Source: CAD feature listing. Evaluate the final solid. Frame: model axes, mm. Face numbers are marked on the shaded views. A direction names the side the tool comes from. Give positions to 0.01 mm unless a question says otherwise; leave off trailing zeros. Loops run counter-clockwise (first coordinate to the right, second up) from the corner with the lowest first, then second, coordinate; pieces in that order, holes last. Notation, with made-up numbers: (47, 41.5) -> (57, 41.5) arc R19 cw to (57, 55.5) -> close; hole circle Ø9 at (-40, 30.25). An arc over 180 degrees is marked (long way). Return JSON: item names as keys, results as strings. Group by question number.
(1) Draft query along Y for the marked faces 1, 2 and 3. Return one class per face: released by +Y, released by -Y, zero draft, split by the parting line, or undercut.
(2) Cut plane A-A on z = 14. Return loops of the section in (x, y), then the cut area to 3 significant figures.
(3) Pin query (flat end, axial travel): pin 1 (4 mm diameter, centred on x = 77, y = 83.5, fed in from -Z); pin 2 (10 mm diameter, centred on x = -167, z = 35.5, fed in from -Y); pin 3 (21 mm diameter, centred on y = -2, z = 13, fed in from -X); pin 4 (3 mm diameter, centred on x = -65, y = -16, fed in from -Z). Return the tip coordinate at first contact, or that it passes through.
(4) Cut plane C-C on x = -182. Return loops of the section in (y, z).
(5) Ray query, line 1 (Y direction, x = 21, z = 6); line 2 (Z direction, x = 36, y = -54); line 3 (Y direction, x = -1, z = 8). Return the intervals inside material, ascending. Write a range as from..to.
(6) Cut plane B-B on x = 12. Return loops of the section in (y, z).
(7) Cut plane D-D on y = 68. Return loops of the section in (x, z), then the cut area to 3 significant figures.
(8) Access query for the marked faces 4, 5 and 6. Directions: +Z, -Z, +X, -X, +Y, -Y. A direction counts if a zero-diameter tool reaches every point of the face in a straight line with its end or side. Return the directions, or none.
```python
from build123d import *

# Parameters (mm, degrees)
SKETCH1_R           = 20
BOSS_EXTRUDE1_DEPTH = 50.8
SKETCH2_R           = 39.05
CUT_EXTRUDE2_DEPTH  = 19.05


with BuildPart() as part:
    # Sketch1 → Boss-Extrude1 (new body)
    with BuildSketch(Plane.XY):
        with BuildLine():
            Line((114.3, 42.12), (114.3, -42.12))
            ThreePointArc((114.3, -42.12), (112.822576646, -59.071852399), (105.83, -74.584813154))
            ThreePointArc((105.83, -74.584813154), (80.699418732, -92.137099347), (52.095309818, -103.156800734))
            ThreePointArc((52.095309818, -103.156800734), (-100.055730281, -94.328415864), (-219.763830855, 0))
            ThreePointArc((-219.763830855, 0), (-220.731129195, 55.788021762), (-169.90706285, 78.813080248))
            ThreePointArc((-169.90706285, 78.813080248), (-134.239730538, 79.543465906), (-101.023628706, 92.558174376))
            ThreePointArc((-101.023628706, 92.558174376), (-52.482772845, 114.165280445), (0, 122.450223109))
            ThreePointArc((0, 122.450223109), (57.719827825, 110.208823216), (103.678545425, 73.205760206))
            ThreePointArc((103.678545425, 73.205760206), (111.571353775, 58.545131543), (114.3, 42.12))
        make_face()
        Circle(SKETCH1_R, mode=Mode.SUBTRACT)
    extrude(amount=BOSS_EXTRUDE1_DEPTH)

    # Sketch2 → Cut-Extrude2 (cut)
    with BuildSketch(Plane.XY.offset(50.8)):
        with BuildLine():
            ThreePointArc((95.25, 42.12), (93.54459611, 52.385707215), (88.61159089, 61.548600129))
            ThreePointArc((88.61159089, 61.548600129), (49.546680931, 93.001203687), (0.484827279, 103.406393597))
            ThreePointArc((0.484827279, 103.406393597), (-47.077685611, 95.898164307), (-91.067836236, 76.316724432))
            ThreePointArc((-91.067836236, 76.316724432), (-130.511957161, 60.861758124), (-172.866914281, 59.994425155))
            ThreePointArc((-172.866914281, 59.994425155), (-204.631955747, 45.603763601), (-204.027394284, 10.73625))
            ThreePointArc((-204.027394284, 10.73625), (-93.297401253, -76.517534674), (47.442310838, -84.683790679))
            ThreePointArc((47.442310838, -84.683790679), (70.618294037, -75.913232441), (91.183680686, -62.088842363))
            ThreePointArc((91.183680686, -62.088842363), (94.722194745, -52.857883684), (95.25, -42.986049939))
            Line((95.25, -42.986049939), (95.25, 42.12))
        make_face()
        Circle(SKETCH2_R, mode=Mode.SUBTRACT)
    cut_extrude2 = extrude(amount=-CUT_EXTRUDE2_DEPTH, mode=Mode.SUBTRACT)

    # Mirror5: Cut-Extrude2 across plane
    add(cut_extrude2.mirror(Plane.XY.offset(25.4)), mode=Mode.SUBTRACT)


solid = part.part
```
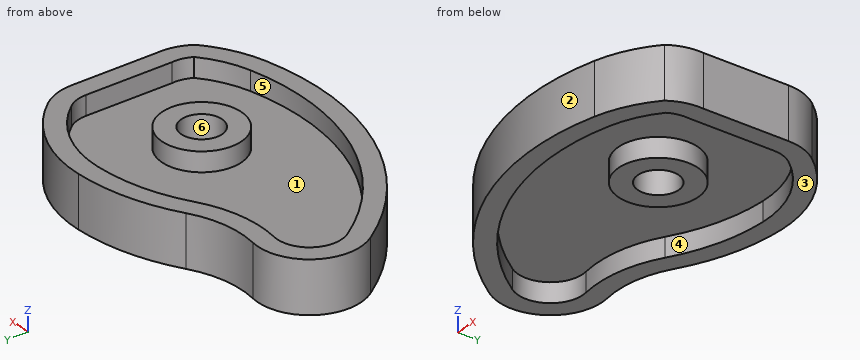
Answers:
{
 "1": {"face 1": "undercut", "face 2": "released by -Y", "face 3": "zero draft"},
 "2": {"outline": "(-219.76, 0) arc R254 ccw to (52.1, -103.16) arc R127 ccw to (105.83, -74.58) arc R50.8 ccw to (114.3, -42.12) -> (114.3, 42.12) arc R50.8 ccw to (103.68, 73.21) arc R127 ccw to (0, 122.45) arc R203.2 ccw to (-101.02, 92.56) arc R101.6 cw to (-169.91, 78.81) arc R50.8 ccw to start; circle Ø78.1 at (0, 0); hole (-204.03, 10.74) arc R234.95 ccw to (47.44, -84.68) arc R107.95 ccw to (91.18, -62.09) arc R31.75 ccw to (95.25, -42.99) -> (95.25, 42.12) arc R31.75 ccw to (88.61, 61.55) arc R107.95 ccw to (0.48, 103.41) arc R184.15 ccw to (-91.07, 76.32) arc R120.65 cw to (-172.87, 59.99) arc R31.75 ccw to start; hole circle Ø40 at (0, 0)", "area": "20,300 mm²"},
 "3": {"pin 1": "z = 0", "pin 2": "y = -60.31", "pin 3": "x = -224.44", "pin 4": "z = 19.05"},
 "4": {"outline": "(-43.7, 0) -> (-16.85, 0) -> (-16.85, 19.05) -> (60.1, 19.05) -> (60.1, 0) -> (79.26, 0) -> (79.26, 50.8) -> (60.1, 50.8) -> (60.1, 31.75) -> (-16.85, 31.75) -> (-16.85, 50.8) -> (-43.7, 50.8) -> close"},
 "5": {"line 1": "-108.96..-89.75, -32.92..32.92, 101.97..121.24", "line 2": "19.05..31.75", "line 3": "-110.69..-91.63, -39.04..-19.97, 19.97..39.04, 103.36..122.42"},
 "6": {"outline": "(-109.9, 0) -> (-90.77, 0) -> (-90.77, 19.05) -> (-37.16, 19.05) -> (-37.16, 0) -> (-16, 0) -> (-16, 50.8) -> (-37.16, 50.8) -> (-37.16, 31.75) -> (-90.77, 31.75) -> (-90.77, 50.8) -> (-109.9, 50.8) -> close; (16, 0) -> (37.16, 0) -> (37.16, 19.05) -> (103.08, 19.05) -> (103.08, 0) -> (122.19, 0) -> (122.19, 50.8) -> (103.08, 50.8) -> (103.08, 31.75) -> (37.16, 31.75) -> (37.16, 50.8) -> (16, 50.8) -> close"},
 "7": {"outline": "(-209.9, 0) -> (-107.26, 0) -> (-107.26, 19.05) -> (83.21, 19.05) -> (83.21, 0) -> (107.21, 0) -> (107.21, 50.8) -> (83.21, 50.8) -> (83.21, 31.75) -> (-107.26, 31.75) -> (-107.26, 50.8) -> (-209.9, 50.8) -> close", "area": "8,850 mm²"},
 "8": {"face 4": "-Z", "face 5": "+Z", "face 6": "+Z, -Z"}
}
